from build123d import *

# Parameters (mm, degrees)
ESBO_O1_R                = 36
RESSALTO_EXTRUS_O1_DEPTH = 150
PADR_O_LINEAR1_COUNT     = 14
PADR_O_LINEAR1_PITCH     = 10
CHANFRO1_SIZE            = 10
ESBO_O4_R                = 22
CORTE_EXTRUS_O1_DEPTH    = 134
ESBO_O5_R                = 1.2
CORTE_EXTRUS_O2_DEPTH    = 134


with BuildPart() as part:
    # Esboço1 → Ressalto-extrusão1 (new body)
    with BuildSketch(Plane.XY):
        Circle(ESBO_O1_R)
    extrude(amount=RESSALTO_EXTRUS_O1_DEPTH)

    # Esboço2 → Corte-Revolução1 (revolve, cut)
    with BuildSketch(Plane(origin=(0, 0, 0), x_dir=(1, 0, 0), z_dir=(0, 1, 0))):
        Polygon((-36, -9.461286074), (-32.715453344, -9.461286074), (-28.965460668, -5.711293398), (-28.965460668, -12.69403838), (-36, -19.728577712), align=None)
    corte_revolu_o1 = revolve(axis=Axis((0, 0, 0), (0, 0, 1)), mode=Mode.SUBTRACT)

    # Padrão linear1: Corte-Revolução1 ×14
    with Locations(*[(0, 0, i * PADR_O_LINEAR1_PITCH) for i in range(1, PADR_O_LINEAR1_COUNT)]):
        add(corte_revolu_o1, mode=Mode.SUBTRACT)

    # Chanfro1
    # the kernel refuses this chamfer: 10 mm, written as the material it takes off along each edge
    with BuildSketch(Plane(origin=(0, 0, 0), x_dir=(1, 0, 0), z_dir=(0, -1, 0))) as chanfro1_piece_1:
        Polygon((36, CHANFRO1_SIZE), (36 - CHANFRO1_SIZE, 0), (36, 0), align=None)
    revolve(axis=Axis((0, 0, 0), (0, 0, 1)), mode=Mode.SUBTRACT)

    # Esboço4 → Corte-extrusão1 (cut)
    with BuildSketch(Plane.XY.offset(150)):
        Circle(ESBO_O4_R)
    extrude(amount=-CORTE_EXTRUS_O1_DEPTH, mode=Mode.SUBTRACT)

    # Esboço5 → Corte-extrusão2 (cut)
    with BuildSketch(Plane.XY.offset(150)):
        with Locations((-27, 0)):
            Circle(ESBO_O5_R)
        with Locations((27, 0)):
            Circle(ESBO_O5_R)
    extrude(amount=-CORTE_EXTRUS_O2_DEPTH, mode=Mode.SUBTRACT)


solid = part.part
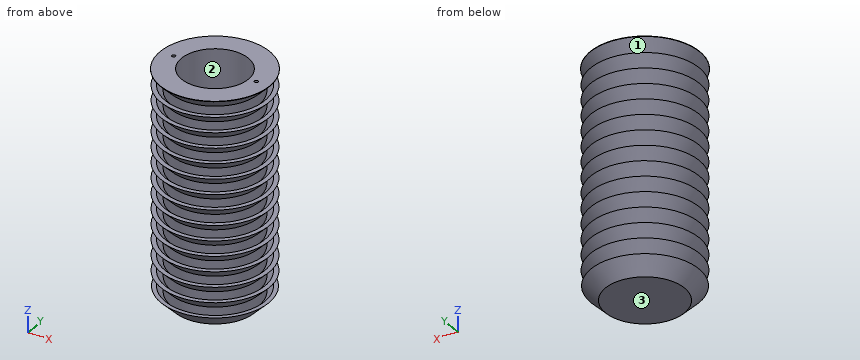
Read the model definition and answer for the solid it produces. Units are mm, in the model's axes. Face numbers are marked on the shaded views. Coordinates: 2 decimals unless noted, no trailing zeros. Order: outer loops, then holes, each group sorted by start corner. A loop starts at its lowest first (then second) coordinate and runs counter-clockwise, first axis right, second up. Notation, with made-up numbers: (-10.5, 52) -> (8.5, 52) arc R18 cw to (8.5, 59) -> close; hole circle Ø6 at (71, 7). An arc over 180 degrees is marked (long way). Answer as a JSON object with one key per item and string values.
1) A cutting plane is placed at B-B, the plane x = 31. State how many separate pieces and enclosed holes the cut face has, plus the area to 3 significant figures.
Model answer:
{"separate pieces": "15", "enclosed holes": "0", "area": "1,340 mm²"}
2) Consider line 1 along X through (y, z) = (9, 48); line 2 along X through (y, z) = (-10, 66); line 3 along Y through (x, z) = (0, 55). Determine where each line is inside the solid, lowest interval first. Write a range as from..to.
Model answer:
{"line 1": "x = -33.07..-29.93, -27.53..-20.07, 20.07..27.53, 29.93..33.07", "line 2": "x = -30.68..-27.49, -27.18..-19.6, 19.6..27.18, 27.49..30.68", "line 3": "y = -31.27..-22, 22..31.27"}
3) The mould has two halves that part along Y. Classify the marked faces 1, 2 and 3: released by +Y, released by -Y, zero draft, split by the parting line, or undercut.
Model answer:
{"face 1": "split by the parting line", "face 2": "undercut", "face 3": "zero draft"}
4) Each of these flat-tipped pins is pushed along its axis until it touches: pin 1 (0.7 mm diameter, centred on x = -27, y = -0.5, fed in from +Z); pin 2 (5 mm diameter, centred on y = 24, z = 62, fed in from +X); pin 3 (4 mm diameter, centred on x = 18, y = 21.5, fed in from -Z). Where does it stop, or does it pass through?
Model answer:
{"pin 1": "stops at z = 16", "pin 2": "stops at x = 20.25", "pin 3": "stops at z = 0.04"}
5) A cutting plane is placed at A-A, the plane z = 138. Determine the outline of the cut face in (x, y), plus the area to 3 significant figures.
Model answer:
{"outline": "circle Ø68.54 at (0, 0); circle Ø57.93 at (0, 0); hole circle Ø62.51 at (0, 0); hole circle Ø2.4 at (-27, 0); hole circle Ø44 at (0, 0); hole circle Ø2.4 at (27, 0)", "area": "1,730 mm²"}
